Build history of the part. All positions in model axes, mm. Face numbers are marked on the shaded views. A direction names the side the tool comes from. Coordinates: 2 decimals unless noted, no trailing zeros. Loops run counter-clockwise (first coordinate to the right, second up) from the corner with the lowest first, then second, coordinate; pieces in that order, holes last. Notation, with made-up numbers: (32, 56) - (38, 56) arc R32 cw to (38, 92) - close; hole circle Ø9 at (30, -2.5). An arc over 180 degrees is marked (long way). One line per item, written item: value.
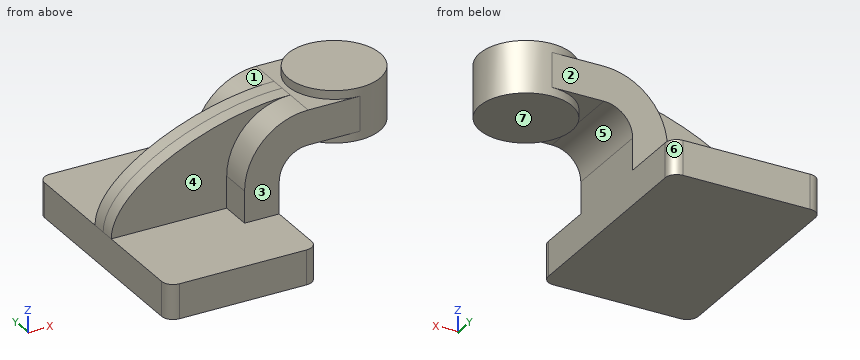
```python
from build123d import *

# Parameters (mm, degrees)
F1_DEPTH = 63.5
F2_DEPTH = 25.4
F3_DEPTH = 7.9375
F0_W     = 25.4
F0_H     = 19.0500000358
F4_DEPTH = 25.4
F6_R     = 6.35


# Not quite as in the source:
# - a feature names something its author has since deleted; it is built from what else it names


with BuildPart() as f1:
    # F0 (on Front) → F1 (new body, symmetric)
    with BuildSketch(Plane.XZ):
        Polygon((-41.275, 9.525), (-41.275, -9.525), (41.275, -9.525), (41.275, 9.525), (22.2249999642, 9.525), align=None)
    extrude(amount=F1_DEPTH, both=True)

    # F0 (on Front) → F2 (join, symmetric)
    with BuildSketch(Plane.XZ):
        with BuildLine():
            Line((22.2249999642, 9.525), (41.275, 9.525))
            Line((41.275, 9.525), (41.275, 27.0002))
            ThreePointArc((41.275, 27.0002), (45.9246798487, 38.2255201513), (57.15, 42.8752))
            Line((57.15, 42.8752), (60.325, 42.8752))
            Line((60.325, 42.8752), (60.325, 61.9252000358))
            Line((60.325, 61.9252000358), (57.15, 61.9252000358))
            ThreePointArc((57.15, 61.9252000358), (32.4542956418, 51.6959043582), (22.2249999642, 27.0002))
            Line((22.2249999642, 27.0002), (22.2249999642, 9.525))
        make_face()
    extrude(amount=F2_DEPTH, both=True)

    # F0 (on Front) → F3 (join, symmetric)
    with BuildSketch(Plane.XZ):
        with BuildLine():
            add(Edge.make_bspline(
                [(-41.275, 9.525), (-41.1172062159, 36.9034484029), (15.5369872227, 62.0494298637), (57.15, 61.9252000358)],
                knots=[0, 0, 0, 0, 111.5045361803, 111.5045361803, 111.5045361803, 111.5045361803], degree=3))
            Line((-41.275, 9.525), (22.2249999642, 9.525))
            Line((22.2249999642, 9.525), (22.2249999642, 27.0002))
            ThreePointArc((22.2249999642, 27.0002), (32.4542956418, 51.6959043582), (57.15, 61.9252000358))
        make_face()
    extrude(amount=F3_DEPTH, both=True)

    # F0 (on Front) → F4 (join, symmetric)
    with BuildSketch(Plane.XZ):
        with Locations((73.025, 52.4002000179)):
            Rectangle(F0_W, F0_H)
    extrude(amount=F4_DEPTH, both=True)

    # F0 (on Front) → F5 (revolve)
    with BuildSketch(Plane.XZ):
        Polygon((85.725, 66.675), (85.725, 61.9252000358), (85.725, 42.8752), (85.725, 38.1), (111.125, 38.1), (111.125, 66.675), align=None)
    revolve(axis=Axis((85.725, 0, 52.3875), (0, 0, 1)))

    # F6
    f6_edges = [f1.edges().sort_by_distance(p)[0] for p in [
        (41.275, -63.5, 0),
        (-41.275, -63.5, 0),
        (41.275, 63.5, 0),
        (-41.275, 63.5, 0),
    ]]
    fillet(f6_edges, radius=F6_R)


solid = f1.part
```
Item 1: Probe probe 1 along Z at (x, y) = (-5, -11) (3 decimals); probe 2 along X at (y, z) = (54, 6) (3 decimals); probe 3 along Y at (x, z) = (79, 60). List the from-to ranges inside material, lowest first. Write a range as from..to.
Check result:
probe 1: z = -9.525..9.525
probe 2: x = -41.275..41.275
probe 3: y = -25.4..25.4
Item 2: Tool access for the marked faces 1, 2, 3 and 4: list every direction of +Z, -Z, +X, -X, +Y, -Y with a clear straight run to the whole face (end or side of a thin tool).
Check result:
face 1: +Z, -X, +Y
face 2: +Z, +X, -X, +Y
face 3: +Z, +X, -X, -Y
face 4: +Z, -X, -Y
Item 3: Cut at C-C, the plane y = -22. Write the cut outline in (x, z) (3 decimals), then the cut area to 3 significant figures.
Check result:
outline: (-41.275, -9.525) - (41.275, -9.525) - (41.275, 27) arc R15.875 cw to (57.15, 42.875) - (73.03, 42.875) - (73.03, 38.1) - (98.42, 38.1) - (98.42, 66.675) - (73.03, 66.675) - (73.03, 61.925) - (57.15, 61.925) arc R34.925 ccw to (22.225, 27) - (22.225, 9.525) - (-41.275, 9.525) - close
area: 3,690 mm^2
Item 4: Cut at D-D, the plane x = 90. Write the cut outline in (y, z) (3 decimals).
Check result:
outline: (-25.038, 38.1) - (25.038, 38.1) - (25.038, 66.675) - (-25.038, 66.675) - close
Item 5: Drop flat-ended pins along their axis: P1, Ø1.5, axis at y = -16.5, z = 58.5, coming from the -X side; P2, Ø14.5, axis at x = 76.5, y = 8.5, coming from the -Z side; P3, Ø11, axis at y = 2, z = 10.5, coming from the +X side (3 decimals). Give the stop position or say it passes through.
Check result:
P1: stops at x = 40.59
P2: stops at z = 38.1
P3: stops at x = 41.275
Item 6: Cut at A-A, the plane y = 17. Write the cut outline in (x, z) (3 decimals).
Check result:
outline: (-41.275, -9.525) - (41.275, -9.525) - (41.275, 27) arc R15.875 cw to (57.15, 42.875) - (66.853, 42.875) - (66.853, 38.1) - (104.597, 38.1) - (104.597, 66.675) - (66.853, 66.675) - (66.853, 61.925) - (57.15, 61.925) arc R34.925 ccw to (22.225, 27) - (22.225, 9.525) - (-41.275, 9.525) - close
Item 7: Pull direction X, two halves, no side cores. Call the marked faces 5, 6 and 7: released by +X, released by -X, zero draft, split by the parting line, or undercut.
Check result:
face 5: undercut
face 6: released by +X
face 7: zero draft
Item 8: Cut at B-B, the plane x = 65. Write the cut outline in (y, z) (1 decimal).
Check result:
outline: (-25.4, 42.9) - (-14.7, 42.9) - (-14.7, 38.1) - (14.7, 38.1) - (14.7, 42.9) - (25.4, 42.9) - (25.4, 61.9) - (14.7, 61.9) - (14.7, 66.7) - (-14.7, 66.7) - (-14.7, 61.9) - (-25.4, 61.9) - close
